Build history of the part. All positions in model axes, mm. A direction names the side the tool comes from. Round coordinates to 2 decimals unless told otherwise and drop trailing zeros. Write each loop counter-clockwise with the first axis right and the second up, starting at its lowest first coordinate (ties: lowest second). Pieces come first, ordered by that corner, then holes. Notation, with made-up numbers: (-33, 58.25) -> (-4, 58.25) arc R32 cw to (-4, 89.25) -> close; hole circle Ø1 at (24, 27). An arc over 180 degrees is marked (long way). One line per question, with ' | ' between items.
Autodesk Inventor part; units mm, degrees
ref_plane "Plano de trabajo1" through (0, -15, 0) normal (0, -1, 0) x (1, 0, 0)
ref_plane "YZ Plane" through (0, 0, 0) normal (1, 0, 0) x (0, 1, 0)
ref_plane "XZ Plane" through (0, 0, 0) normal (0, 1, 0) x (-1, 0, 0)
sketch "Boceto1" plane through (0, 0, 0) normal (0, 1, 0) x (-1, 0, 0)
  line L0 (21.15, 21.15) -> (-21.15, 21.15)
  line L1 (-21.15, 21.15) -> (-21.15, -21.15)
  line L2 (-21.15, -21.15) -> (21.15, -21.15)
  line L3 (21.15, -21.15) -> (21.15, 21.15)
  line L4 (0, 0) -> (3.2885, 0)
  line L5 (0, 0) -> (0, -4.7563)
  circle A0 centre (0, 0) radius 7.5
  line L6 (21.15, -21.15) -> (35, -21.15)
  line L7 (35, -21.15) -> (35, 21.15)
  line L8 (35, 21.15) -> (21.15, 21.15)
  line L9 (21.15, 21.15) -> (21.15, -21.15)
  dimension "d0" = 42.3
  dimension "d1" = 42.3
  dimension "d26" = 15
  dimension "d35" = 35
extrude "Extrusión1" add sketch "Boceto1" along normal blind 5
sketch "Boceto2" plane through (0, 5, 0) normal (0, 1, 0) x (1, 0, 0)
  circle A0 centre (-15.5, 15.5) radius 1.5
  point P0 (0, 0)
  dimension "d4" = 3
  dimension "d5" = 15.5
  dimension "d6" = 15.5
extrude "Extrusión2" cut sketch "Boceto2" against normal through all
pattern_circular "Patrón circular1" count 4 over 360 about axis through (0, -10, 0) along (0, 1, 0) of "Extrusión2"
sketch "Boceto7" plane through (0, 0, 0) normal (0, -1, 0) x (1, 0, 0)
  circle A0 centre (-26.3, 0) radius 2
  point P0 (0, 0)
  dimension "d31" = 4
  dimension "d32" = 26.3
extrude "Extrusión7" cut sketch "Boceto7" against normal through all
sketch "Boceto8" plane through (21.15, 0, -21.15) normal (0, 0, -1) x (-1, 0, 0)
  line L0 (0, 0) -> (0, 5)
  line L1 (0, 0) -> (56.15, 0)
  line L2 (56.15, 0) -> (56.15, 44)
  line L3 (56.15, 44) -> (0, 44)
  line L4 (0, 44) -> (0, 0)
  line L5 (0, 5) -> (56.15, 5)
  point P0 (21.15, 0)
  dimension "d36" = 39
extrude "Extrusión8" add sketch "Boceto8" along normal blind 5
ref_plane "Plano de trabajo1" through (0, -15, 0) normal (0, -1, 0) x (1, 0, 0)
sketch "Boceto9" plane through (0, -15, 0) normal (0, -1, 0) x (1, 0, 0)
  line L0 (21.15, 21.15) -> (21.15, -26.15)
  line L1 (-35, 21.15) -> (21.15, 21.15)
  line L2 (-35, 21.15) -> (-35, -26.15)
  circle A0 centre (0, 0) radius 2.5
  circle A1 centre (-26.3, 0) radius 2
  line L3 (-35, -21.15) -> (-35, 21.15)
  line L4 (21.15, -26.15) -> (-35, -26.15)
  line L5 (-35, -26.15) -> (-35, -8.65)
  line L6 (-35, -8.65) -> (21.15, -8.65)
  line L7 (21.15, -8.65) -> (21.15, -26.15)
  point P0 (-35, -26.15)
  point P1 (21.15, -8.65)
  dimension "d45" = 5
  dimension "d46" = 17.5
extrude "Extrusión9" add sketch "Boceto9" along normal blind 5 contours L0 L6 L2 L1
sketch "Boceto10" plane through (0, -20, 0) normal (0, -1, 0) x (1, 0, 0)
  line L0 (-35, -8.65) -> (21.15, -8.65)
  line L1 (21.15, -8.65) -> (26.15, -8.65)
  line L2 (26.15, -8.65) -> (26.15, 26.15)
  line L3 (26.15, 26.15) -> (-40, 26.15)
  line L4 (-40, 26.15) -> (-40, -8.65)
  line L5 (-40, -8.65) -> (-35, -8.65)
  line L6 (-35, -21.15) -> (-35, 21.15)
  line L7 (21.15, 21.15) -> (-35, 21.15)
  line L8 (21.15, -8.65) -> (21.15, 21.15)
  line L9 (-35, 21.15) -> (-35, -8.65)
  point P0 (0, 0)
  dimension "d47" = 5
  dimension "d48" = 5
  dimension "d49" = 5
extrude "Extrusión10" add sketch "Boceto10" against normal up to surface (25 mm away) contours L5 L4 L3 L2 L1 L8 L7 L6
equation "\"d0\" = d1"
equation "\"d48\" = d47"
equation "\"d49\" = d47"
properties part number "Base Motor X1"
(1) Wall check: line 1 (X direction, y = 1.75, z = -15.5); line 2 (Y direction, x = -29.5, z = 0.5); line 3 (Z direction, x = -15.5, y = 1.7). Give the ranges that are in metal, low to high. Write a range as from..to.
Calculated:
line 1: -35..-17, -14..14, 17..21.15 | line 2: -20..-15, 0..5 | line 3: -26.15..-17, -14..14, 17..26.15
(2) Mould opens along X. For faces 5 (the flat face through (21.15, 17, -23)), 6 (the flat face through (-35, -8, 6)), 7 (the flat face through (-7, -16, -8.65)) say: pulls with the +X half, pulls with the -X half, needs draft (parallel to the pull), parting line crosses it, or undercut.
Calculated:
face 5: pulls with the +X half | face 6: undercut | face 7: needs draft
(3) Slice it at A-A (x = 0). Write the cut outline in (y, z), then the cut area to 4 significant figures.
Calculated:
outline: (-20, -8.65) -> (-15, -8.65) -> (-15, -2.5) -> (-20, -2.5) -> close; (-20, 2.5) -> (-15, 2.5) -> (-15, 21.15) -> (0, 21.15) -> (0, 7.5) -> (5, 7.5) -> (5, 26.15) -> (-20, 26.15) -> close; (0, -26.15) -> (44, -26.15) -> (44, -21.15) -> (5, -21.15) -> (5, -7.5) -> (0, -7.5) -> close | area: 605.5 mm2
(4) Slice it at D-D (z = 9). Write the cut outline in (x, y), then the cut area to 4 significant figures.
Calculated:
outline: (-40, -20) -> (26.15, -20) -> (26.15, 5) -> (-40, 5) -> close; hole (-35, -15) -> (21.15, -15) -> (21.15, 0) -> (-35, 0) -> close | area: 811.5 mm2
(5) 3-axis set-ups, long thin cutter, end or side, ignore diameter. For faces 1 (the flat face through (-7, 25, -21.15)), 2 (the flat face through (21.15, -8, 6)), 3 (the cylindrical face through (7.493, 2.465, -0.33)), 4 (the flat face through (-6, -8, 26.15)): which of +Z, -Z, +X, -X, +Y, -Y reach the whole face in a straight line?
Calculated:
face 1: +Z, +X, -X, +Y | face 2: -Z | face 3: +Y | face 4: +Z, +X, -X, +Y, -Y
(6) Slice it at B-B (z = 15.5). Write the cut outline in (x, y), then the cut area to 4 significant figures.
Calculated:
outline: (-40, -20) -> (26.15, -20) -> (26.15, 5) -> (17, 5) -> (17, 0) -> (21.15, 0) -> (21.15, -15) -> (-35, -15) -> (-35, 0) -> (-17, 0) -> (-17, 5) -> (-40, 5) -> close; (-14, 0) -> (14, 0) -> (14, 5) -> (-14, 5) -> close | area: 781.5 mm2
(7) Drop flat-ended pins along their axis: pin 1 (1.5 mm diameter, centred on x = -29, y = 22.5, fed in from +Z); pin 2 (3 mm diameter, centred on x = -31.5, z = -19.5, fed in from +Y); pin 3 (12 mm diameter, centred on x = -14, y = -10.5, fed in from -Z); pin 4 (12 mm diameter, centred on y = 11.5, z = -1, fed in from -X). Give the stop position or say it passes through.
Calculated:
pin 1: z = -21.15 | pin 2: y = 5 | pin 3: z = -8.65 | pin 4: through
(8) Slice it at C-C (z = -15.5). Write the cut outline in (x, y), then the cut area to 3 significant figures.
Calculated:
outline: (-35, 0) -> (-17, 0) -> (-17, 5) -> (-35, 5) -> close; (-14, 0) -> (14, 0) -> (14, 5) -> (-14, 5) -> close; (17, 0) -> (21.15, 0) -> (21.15, 5) -> (17, 5) -> close | area: 251 mm2
